Build history of the part. All positions in model axes, mm. A direction names the side the tool comes from. Give positions to 0.01 mm unless a question says otherwise; leave off trailing zeros. Put each result on its own line as item: value.
```python
from build123d import *

# Parameters (mm, degrees)
F0_W     = 500
F0_H     = 20
F1_DEPTH = 4.5
F2_DEPTH = 6.1
F3_D     = 13


with BuildPart() as f1:
    # F0 (on Top) → F1 (new body)
    with BuildSketch(Plane.XY):
        with Locations((0, 340)):
            Rectangle(F0_W, F0_H)
    extrude(amount=F1_DEPTH)



with BuildPart() as f1b:
    # F0 (on Top) → F1, piece 2 (new body)
    with BuildSketch(Plane.XY):
        with Locations((0, 300)):
            Rectangle(F0_W, F0_H)
    extrude(amount=F1_DEPTH)


with BuildPart() as f1c:
    # F0 (on Top) → F1, piece 3 (new body)
    with BuildSketch(Plane.XY):
        with Locations((0, 260)):
            Rectangle(F0_W, F0_H)
    extrude(amount=F1_DEPTH)


with BuildPart() as f1d:
    # F0 (on Top) → F1, piece 4 (new body)
    with BuildSketch(Plane.XY):
        with Locations((0, 220)):
            Rectangle(F0_W, F0_H)
    extrude(amount=F1_DEPTH)


with BuildPart() as f1e:
    # F0 (on Top) → F1, piece 5 (new body)
    with BuildSketch(Plane.XY):
        with Locations((0, 180)):
            Rectangle(F0_W, F0_H)
    extrude(amount=F1_DEPTH)


with BuildPart() as f1f:
    # F0 (on Top) → F1, piece 6 (new body)
    with BuildSketch(Plane.XY):
        with Locations((0, 140)):
            Rectangle(F0_W, F0_H)
    extrude(amount=F1_DEPTH)


with BuildPart() as f1g:
    # F0 (on Top) → F1, piece 7 (new body)
    with BuildSketch(Plane.XY):
        with Locations((0, 100)):
            Rectangle(F0_W, F0_H)
    extrude(amount=F1_DEPTH)


with BuildPart() as f1h:
    # F0 (on Top) → F1, piece 8 (new body)
    with BuildSketch(Plane.XY):
        with Locations((0, 60)):
            Rectangle(F0_W, F0_H)
    extrude(amount=F1_DEPTH)


with BuildPart() as f1i:
    # F0 (on Top) → F1, piece 9 (new body)
    with BuildSketch(Plane.XY):
        with Locations((0, 20)):
            Rectangle(F0_W, F0_H)
    extrude(amount=F1_DEPTH)


with BuildPart() as f1j:
    # F0 (on Top) → F1, piece 10 (new body)
    with BuildSketch(Plane.XY):
        with Locations((0, -20)):
            Rectangle(F0_W, F0_H)
    extrude(amount=F1_DEPTH)


with BuildPart() as f1k:
    # F0 (on Top) → F1, piece 11 (new body)
    with BuildSketch(Plane.XY):
        with Locations((0, -60)):
            Rectangle(F0_W, F0_H)
    extrude(amount=F1_DEPTH)


with BuildPart() as f1l:
    # F0 (on Top) → F1, piece 12 (new body)
    with BuildSketch(Plane.XY):
        with Locations((0, -100)):
            Rectangle(F0_W, F0_H)
    extrude(amount=F1_DEPTH)


with BuildPart() as f1m:
    # F0 (on Top) → F1, piece 13 (new body)
    with BuildSketch(Plane.XY):
        with Locations((0, -140)):
            Rectangle(F0_W, F0_H)
    extrude(amount=F1_DEPTH)


with BuildPart() as f1n:
    # F0 (on Top) → F1, piece 14 (new body)
    with BuildSketch(Plane.XY):
        with Locations((0, -180)):
            Rectangle(F0_W, F0_H)
    extrude(amount=F1_DEPTH)


with BuildPart() as f1o:
    # F0 (on Top) → F1, piece 15 (new body)
    with BuildSketch(Plane.XY):
        with Locations((0, -220)):
            Rectangle(F0_W, F0_H)
    extrude(amount=F1_DEPTH)


with BuildPart() as f1p:
    # F0 (on Top) → F1, piece 16 (new body)
    with BuildSketch(Plane.XY):
        with Locations((0, -260)):
            Rectangle(F0_W, F0_H)
    extrude(amount=F1_DEPTH)


with BuildPart() as f1q:
    # F0 (on Top) → F1, piece 17 (new body)
    with BuildSketch(Plane.XY):
        with Locations((0, -300)):
            Rectangle(F0_W, F0_H)
    extrude(amount=F1_DEPTH)


with BuildPart() as f1r:
    # F0 (on Top) → F1, piece 18 (new body)
    with BuildSketch(Plane.XY):
        with Locations((0, -340)):
            Rectangle(F0_W, F0_H)
    extrude(amount=F1_DEPTH)


with BuildPart() as f1_1:
    add(f1.part)

    add(f1b.part)  # F2 merges F1b

    add(f1c.part)  # F2 merges F1c

    add(f1d.part)  # F2 merges F1d

    add(f1e.part)  # F2 merges F1e

    add(f1f.part)  # F2 merges F1f

    add(f1g.part)  # F2 merges F1g

    add(f1h.part)  # F2 merges F1h

    add(f1i.part)  # F2 merges F1i

    add(f1j.part)  # F2 merges F1j

    add(f1k.part)  # F2 merges F1k

    add(f1l.part)  # F2 merges F1l

    add(f1m.part)  # F2 merges F1m

    add(f1n.part)  # F2 merges F1n

    add(f1o.part)  # F2 merges F1o

    add(f1p.part)  # F2 merges F1p

    add(f1q.part)  # F2 merges F1q

    add(f1r.part)  # F2 merges F1r
    # F0 (on Top) → F2 (join)
    with BuildSketch(Plane.XY):
        with Locations((0, 320)):
            Rectangle(F0_W, F0_H)
        with Locations((0, 280)):
            Rectangle(F0_W, F0_H)
        with Locations((0, 240)):
            Rectangle(F0_W, F0_H)
        with Locations((0, 200)):
            Rectangle(F0_W, F0_H)
        with Locations((0, 160)):
            Rectangle(F0_W, F0_H)
        with Locations((0, 120)):
            Rectangle(F0_W, F0_H)
        with Locations((0, 80)):
            Rectangle(F0_W, F0_H)
        with Locations((0, 40)):
            Rectangle(F0_W, F0_H)
        Rectangle(F0_W, F0_H)
        with Locations((0, -40)):
            Rectangle(F0_W, F0_H)
        with Locations((0, -80)):
            Rectangle(F0_W, F0_H)
        with Locations((0, -120)):
            Rectangle(F0_W, F0_H)
        with Locations((0, -160)):
            Rectangle(F0_W, F0_H)
        with Locations((0, -200)):
            Rectangle(F0_W, F0_H)
        with Locations((0, -240)):
            Rectangle(F0_W, F0_H)
        with Locations((0, -280)):
            Rectangle(F0_W, F0_H)
        with Locations((0, -320)):
            Rectangle(F0_W, F0_H)
    extrude(amount=F2_DEPTH)

    # F3 (through all)
    with Locations(Plane(origin=(0, 0, 0), x_dir=(1, 0, 0), z_dir=(0, 0, -1))):
        with Locations((0, -325), (0, -275)):
            Hole(F3_D / 2)


solid = f1_1.part
```
Q1. Probe line 1 (Y direction, x = 0, z = 1.5); line 2 (X direction, y = 275, z = 3); line 3 (Z direction, x = -155.5, y = -148). List the from-to ranges inside material, lowest first. Write a range as from..to.
Here are the results:
line 1: -350..268.5, 281.5..318.5, 331.5..350
line 2: -250..-6.5, 6.5..250
line 3: 0..4.5
Q2. Tool access for faces 1 (the flat face through (-3, -60, 4.5)), 2 (the flat face through (-3, 340, 4.5)), 3 (the flat face through (-3, -340, 4.5)): list every direction of +Z, -Z, +X, -X, +Y, -Y with a clear straight run to the whole face (end or side of a thin tool).
Here are the results:
face 1: +Z, +X, -X
face 2: +Z, +X, -X, +Y
face 3: +Z, +X, -X, -Y
Q3. Drop flat-ended pins along their axis: pin 1 Ø10 at (x, y) = (-15.5, -221) entering from +Z; pin 2 Ø1.3 at (x, z) = (76.5, 5.5) entering from -Y; pin 3 Ø0.8 at (x, z) = (38, 5.5) entering from +Y. Give the stop position or say it passes through.
Here are the results:
pin 1: z = 4.5
pin 2: y = -330
pin 3: y = 330
Q4. Mould opens along Y. For faces 4 (the flat face through (-3, 0, 6.1)), 5 (the flat face through (-3, -140, 4.5)) say: pulls with the +Y half, pulls with the -Y half, needs draft (parallel to the pull), parting line crosses it, or undercut.
Here are the results:
face 4: needs draft
face 5: undercut
